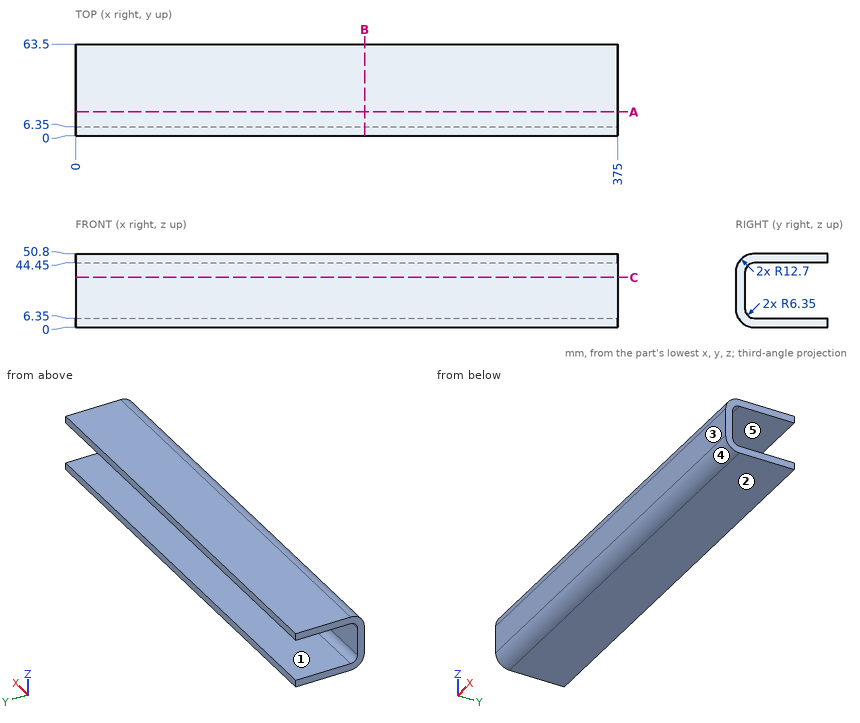
Can you work these out from the drawing? Everything is in mm from the part's minimum corner. A direction names the side the tool comes from. Coordinates: 2 decimals unless noted, no trailing zeros. Loops run counter-clockwise (first coordinate to the right, second up) from the corner with the lowest first, then second, coordinate; pieces in that order, holes last.
1. If we mould it in two halves opening along Z, with no side actions, what happens to the marked faces 1, 2 and 3? For each: pulls with the +Z half, pulls with the -Z half, needs draft (parallel to the pull), parting line crosses it, or undercut.
2. I need wall thicknesses on L1, parallel to Z at x = 49.5, y = 17; L2, parallel to Y at x = 129, z = 14; L3, parallel to Z at x = 283.5, y = 7. Which ranges of each line are inside material? Lowest first, please.
3. For P1, Ø1, axis at x = 312.5, z = 13, coming from the +Y side; P2, Ø5, axis at x = 218, y = 6.5, coming from the +Z side, each with a flat end and sliding along its axis, tell me the tip position at first contact or that it passes through.
4. Imagine slicing it at C-C, the plane z = 34.5. Please give me the cut outline in (x, y).
5. Imagine slicing it at B-B, the plane x = 200. Please give me the cut outline in (y, z), and give its area (3 significant figures).
6. For the marked faces 4 and 5, which set-ups out of +Z, -Z, +X, -X, +Y, -Y let a thin tool reach every point of the face, with its end or its side?
7. Imagine slicing it at A-A, the plane y = 16.5. Please give me the cut outline in (x, z), and give its area (3 significant figures).
Taken from the geometry:
1. face 1: undercut
1. face 2: pulls with the -Z half
1. face 3: needs draft
2. L1: z = 0 to 6.35, 44.45 to 50.8
2. L2: y = 0 to 6.35
2. L3: z = 1.35 to 9.9, 40.9 to 49.45
3. P1: stops at y = 6.35
3. P2: stops at z = 50.25
4. outline: (0, 0) - (375, 0) - (375, 6.35) - (0, 6.35) - close
5. outline: (0, 12.7) arc R12.7 ccw to (12.7, 0) - (63.5, 0) - (63.5, 6.35) - (12.7, 6.35) arc R6.35 cw to (6.35, 12.7) - (6.35, 38.1) arc R6.35 cw to (12.7, 44.45) - (63.5, 44.45) - (63.5, 50.8) - (12.7, 50.8) arc R12.7 ccw to (0, 38.1) - close
5. area: 996 mm2
6. face 4: -Z, +X, -X, -Y
6. face 5: +X, -X, +Y
7. outline: (0, 0) - (375, 0) - (375, 6.35) - (0, 6.35) - close; (0, 44.45) - (375, 44.45) - (375, 50.8) - (0, 50.8) - close
7. area: 4,760 mm2
